Can you work these out from the model? Positions are in its coordinate system, mm. Face numbers are marked on the shaded views. Give positions to 0.01 mm unless a question says otherwise; leave off trailing zeros. Write each loop counter-clockwise with the first axis right and the second up, starting at its lowest first coordinate (ties: lowest second). Pieces come first, ordered by that corner, then holes. Notation, with made-up numbers: (33.25, 44.5) - (50.25, 44.5) arc R26 ccw to (50.25, 80.5) - close; hole circle Ø10 at (-0.5, 55.25). An arc over 180 degrees is marked (long way). Return JSON: item names as keys, results as strings. Group by question number.
from build123d import *

# Parameters (mm, degrees)
SKETCH1_W              = 29
SKETCH1_H              = 8
BOSS_EXTRUDE1_DEPTH    = 3
M2_5_CLEARANCE_HOLE1_D = 2.9
FILLET1_R              = 3


with BuildPart() as part:
    # Sketch1 → Boss-Extrude1 (new body)
    with BuildSketch(Plane(origin=(0, 0, 0), x_dir=(1, 0, 0), z_dir=(0, 1, 0))):
        with Locations((14.5, 4)):
            Rectangle(SKETCH1_W, SKETCH1_H)
    extrude(amount=BOSS_EXTRUDE1_DEPTH)

    # M2.5 Clearance Hole1 (through all)
    with Locations(Plane(origin=(0, 3, 0), x_dir=(1, 0, 0), z_dir=(0, 1, 0))):
        with Locations((6, 4), (23, 4)):
            Hole(M2_5_CLEARANCE_HOLE1_D / 2)

    # Fillet1
    fillet1_edges = [part.edges().sort_by_distance(p)[0] for p in [
        (0, 1.5, -8),
        (29, 1.5, -8),
        (29, 1.5, 0),
        (0, 1.5, 0),
    ]]
    fillet(fillet1_edges, radius=FILLET1_R)


solid = part.part
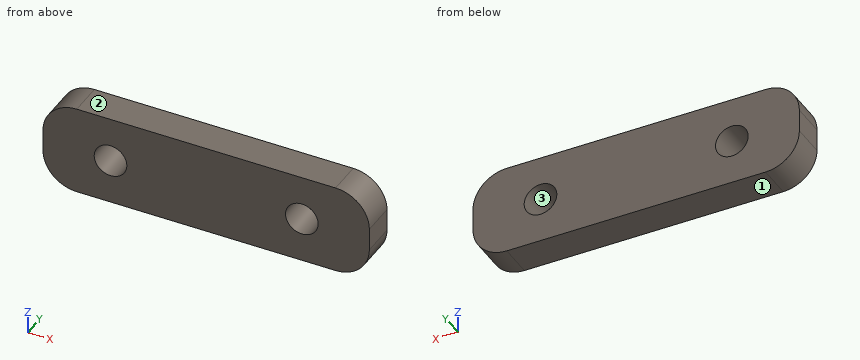
1) I need wall thicknesses on line 1 along X through (y, z) = (1, -5); line 2 along Z through (x, y) = (23, 2.2); line 3 along X through (y, z) = (1.75, -4.75). Which ranges of each line are inside material? Lowest first, please.
2) Imagine slicing it at A-A, the plane y = 1.7. Write out the boundary of the cut face in (x, z), and give its area (3 significant figures).
3) We'd pull the mould along Z, two halves only. Please class the marked faces 1, 2 and 3: pulls with the +Z half, pulls with the -Z half, needs draft (parallel to the pull), parting line crosses it, or undercut.
4) Imagine slicing it at B-B, the plane x = 6. Write out the boundary of the cut face in (y, z), and give its area (3 significant figures).
5) Imagine slicing it at C-C, the plane z = -4. Write out the boundary of the cut face in (x, y), and give its area (3 significant figures).
6) Will this pin go through, and if not, where does the flat tip stop? pin 1 Ø2.5 at (x, z) = (6, -4) entering from +Y.
7) Imagine slicing it at D-D, the plane z = -1.5. Write out the boundary of the cut face in (x, y).
Resolved:
{
 "1": {"line 1": "0 to 4.95, 7.05 to 21.95, 24.05 to 29", "line 2": "-8 to -5.45, -2.55 to 0", "line 3": "0 to 4.76, 7.24 to 21.76, 24.24 to 29"},
 "2": {"outline": "(0, -5) arc R3 ccw to (3, -8) - (26, -8) arc R3 ccw to (29, -5) - (29, -3) arc R3 ccw to (26, 0) - (3, 0) arc R3 ccw to (0, -3) - close; hole circle Ø2.9 at (6, -4); hole circle Ø2.9 at (23, -4)", "area": "211 mm^2"},
 "3": {"face 1": "pulls with the -Z half", "face 2": "pulls with the +Z half", "face 3": "undercut"},
 "4": {"outline": "(0, -8) - (3, -8) - (3, -5.45) - (0, -5.45) - close; (0, -2.55) - (3, -2.55) - (3, 0) - (0, 0) - close", "area": "15.3 mm^2"},
 "5": {"outline": "(0, 0) - (4.55, 0) - (4.55, 3) - (0, 3) - close; (7.45, 0) - (21.55, 0) - (21.55, 3) - (7.45, 3) - close; (24.45, 0) - (29, 0) - (29, 3) - (24.45, 3) - close", "area": "69.6 mm^2"},
 "6": {"pin 1": "through"},
 "7": {"outline": "(0.4, 0) - (28.6, 0) - (28.6, 3) - (0.4, 3) - close"}
}
